Part model, mm, in its own coordinate system. Give positions to 0.01 mm unless a question says otherwise; leave off trailing zeros. Order: outer loops, then holes, each group sorted by start corner. A loop starts at its lowest first (then second) coordinate and runs counter-clockwise, first axis right, second up.
from build123d import *

# Parameters (mm, degrees)
SKETCH1_W           = 130
SKETCH1_H           = 180
BOSS_EXTRUDE1_DEPTH = 6
SKETCH2_R           = 32.5
SKETCH2_W           = 28
SKETCH2_H           = 70
CUT_EXTRUDE2_DEPTH  = 6
SKETCH3_W           = 20
SKETCH3_H           = 49.5
CUT_EXTRUDE3_DEPTH  = 223.117086241
SKETCH4_W           = 44
SKETCH4_H           = 6
SKETCH4_W_2         = 4
SKETCH4_H_2         = 27
CUT_EXTRUDE4_DEPTH  = 223.117086241


with BuildPart() as part:
    # Sketch1 → Boss-Extrude1 (new body)
    with BuildSketch(Plane(origin=(0, 0, 0), x_dir=(1, 0, 0), z_dir=(0, 1, 0))):
        with Locations((65, 90)):
            Rectangle(SKETCH1_W, SKETCH1_H)
    extrude(amount=BOSS_EXTRUDE1_DEPTH)

    # Sketch2 → Cut-Extrude2 (cut)
    with BuildSketch(Plane(origin=(0, 6, 0), x_dir=(1, 0, 0), z_dir=(0, 1, 0))):
        with Locations(Location((65, 41, 0), (0, 0, 270))):
            Circle(SKETCH2_R)
        with Locations((20, 139)):
            Rectangle(SKETCH2_W, SKETCH2_H)
        with Locations((110, 139)):
            Rectangle(SKETCH2_W, SKETCH2_H)
    extrude(amount=-CUT_EXTRUDE2_DEPTH, mode=Mode.SUBTRACT)

    # Sketch3 → Cut-Extrude3 (cut, through all)
    with BuildSketch(Plane(origin=(0, 6, 0), x_dir=(1, 0, 0), z_dir=(0, 1, 0))):
        with Locations((120, 75.25)):
            Rectangle(SKETCH3_W, SKETCH3_H)
        with Locations((10, 75.25)):
            Rectangle(SKETCH3_W, SKETCH3_H)
    extrude(amount=-CUT_EXTRUDE3_DEPTH, mode=Mode.SUBTRACT)

    # Sketch4 → Cut-Extrude4 (cut, through all)
    with BuildSketch(Plane(origin=(0, 6, 0), x_dir=(1, 0, 0), z_dir=(0, 1, 0))):
        with Locations((65, 177)):
            Rectangle(SKETCH4_W, SKETCH4_H)
        with Locations((36, 140.5)):
            Rectangle(SKETCH4_W_2, SKETCH4_H_2)
        with Locations((94, 140.5)):
            Rectangle(SKETCH4_W_2, SKETCH4_H_2)
        with Locations((65, 3)):
            Rectangle(SKETCH4_W, SKETCH4_H)
    extrude(amount=-CUT_EXTRUDE4_DEPTH, mode=Mode.SUBTRACT)


solid = part.part
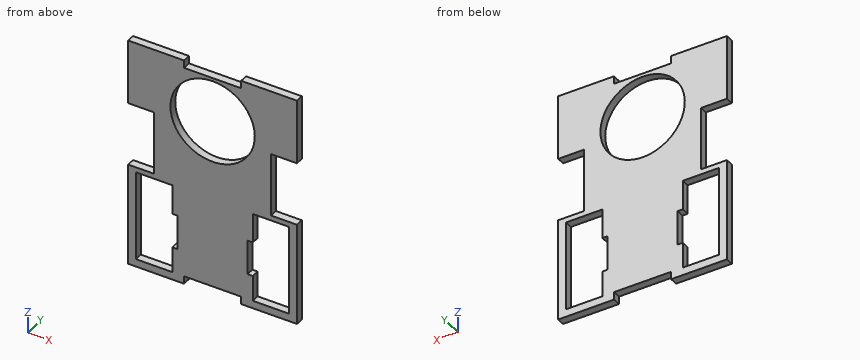
Item 1: Drill centre lines: probe 1 along Z at (x, y) = (6.5, 1.55); probe 2 along X at (y, z) = (1.7, -162.5); probe 3 along X at (y, z) = (3.65, -146.5). Where is each one in solid material? Low to high.
Item 2: Band-saw the part on A-A on x = 65. List the corners of the cut face in (y, z), plus the area to 3 significant figures.
Item 3: Drop flat-ended pins along their axis: P1, Ø1.8, axis at x = 66.5, y = 2, coming from the +Z side; P2, Ø1.5, axis at x = 82.5, y = 3.5, coming from the -Z side. Give the stop position or say it passes through.
Item 4: Band-saw the part on C-C on x = 12. List the corners of the cut face in (y, z).
Item 5: Band-saw the part on B-B on z = -41. List the corners of the cut face in (x, y).
Item 6: Band-saw the part on D-D on z = -124. List the corners of the cut face in (x, y), plus the area to 3 significant figures.
Working result:
1. probe 1: z = -180 to -174, -104 to -100, -50.5 to 0
1. probe 2: x = 0 to 6, 34 to 96, 124 to 130
1. probe 3: x = 0 to 6, 38 to 92, 124 to 130
2. outline: (0, -174) - (6, -174) - (6, -73.5) - (0, -73.5) - close; (0, -8.5) - (6, -8.5) - (6, -6) - (0, -6) - close
2. area: 618 mm2
3. P1: stops at z = -6
3. P2: stops at z = -174
4. outline: (0, -180) - (6, -180) - (6, -174) - (0, -174) - close; (0, -104) - (6, -104) - (6, -100) - (0, -100) - close; (0, -50.5) - (6, -50.5) - (6, 0) - (0, 0) - close
5. outline: (0, 0) - (32.5, 0) - (32.5, 6) - (0, 6) - close; (97.5, 0) - (130, 0) - (130, 6) - (97.5, 6) - close
6. outline: (0, 0) - (6, 0) - (6, 6) - (0, 6) - close; (34, 0) - (96, 0) - (96, 6) - (34, 6) - close; (124, 0) - (130, 0) - (130, 6) - (124, 6) - close
6. area: 444 mm2
